Build history of the part. All positions in model axes, mm. Give positions to 0.01 mm unless a question says otherwise; leave off trailing zeros. Loops run counter-clockwise (first coordinate to the right, second up) from the corner with the lowest first, then second, coordinate; pieces in that order, holes last. Notation, with made-up numbers: (45, -34.75) -> (81, -34.75) arc R28 cw to (81, 2.25) -> close; hole circle Ø1 at (-22.75, 80.5). An arc over 180 degrees is marked (long way). Answer as a JSON object with one key per item and string values. Group by question number.
from build123d import *

# Parameters (mm, degrees)
SKETCH1_W                 = 50
SKETCH1_H                 = 8
BOSS_EXTRUDE1_DEPTH       = 3
F_8_CLEARANCE_HOLE1_D     = 4.4958
F_8_CLEARANCE_HOLE1_DEPTH = 17
F_8_CLEARANCE_HOLE1_TIP   = 1.350674586


with BuildPart() as part:
    # Sketch1 → Boss-Extrude1 (new body)
    with BuildSketch(Plane(origin=(0, 0, 0), x_dir=(1, 0, 0), z_dir=(0, 1, 0))):
        with Locations((17.773632998, 0.313559322)):
            Rectangle(SKETCH1_W, SKETCH1_H)
    extrude(amount=BOSS_EXTRUDE1_DEPTH)

    # #8 Clearance Hole1
    with Locations(Plane(origin=(7.773632998, 3, -0.313559322), x_dir=(0, 0, 1), z_dir=(0, 1, 0))):
        with Locations((0, 0), (0, 20), (0, 10)):
            Hole(F_8_CLEARANCE_HOLE1_D / 2, depth=F_8_CLEARANCE_HOLE1_DEPTH)
            with Locations((0, 0, -(F_8_CLEARANCE_HOLE1_DEPTH + F_8_CLEARANCE_HOLE1_TIP / 2))):  # 118° drill point
                Cone(0, F_8_CLEARANCE_HOLE1_D / 2, F_8_CLEARANCE_HOLE1_TIP, mode=Mode.SUBTRACT)


solid = part.part
(1) Pin check, flat tip, straight feed: pin 1 (1 mm diameter, centred on x = 7.5, z = -1.5, fed in from -Y). Stop position of the tip, or through.
(2) Saw through at B-B on x = 6. List the corners of the cut face in (y, z).
(3) Probe line 1 along X through (y, z) = (0.7, -0.25); line 2 along X through (y, z) = (0.85, -2); line 3 along Z through (x, y) = (27.5, 1.35). List the from-to ranges inside material, lowest first. Write a range as [from, to].
(4) Saw through at A-A on z = -1.5. List the corners of the cut face in (x, y).
(5) Saw through at D-D on z = 1. List the corners of the cut face in (x, y).
(6) Pull direction Z, two halves, no side cores. Call faces 1 (the flat face through (17, 1, -4.314)), 2 (the cylindrical face through (5.58, 1.48, 0.17)), 3 (the flat face through (17, 1, 3.686)), 4 (the flat face through (17, 3, -3)): pulls with the +Z half, pulls with the -Z half, needs draft (parallel to the pull), parting line crosses it, or undercut.
(7) Saw through at C-C on y = 2.05. List the corners of the cut face in (x, z), plus the area to 3 significant figures.
Calculated:
{
 "1": {"pin 1": "passes through"},
 "2": {"outline": "(0, -4.31) -> (3, -4.31) -> (3, -1.69) -> (0, -1.69) -> close; (0, 1.07) -> (3, 1.07) -> (3, 3.69) -> (0, 3.69) -> close"},
 "3": {"line 1": "x = [-7.23, 5.53], [10.02, 15.53], [20.02, 25.53], [30.02, 42.77]", "line 2": "x = [-7.23, 6.29], [9.26, 16.29], [19.26, 26.29], [29.26, 42.77]", "line 3": "z = [-4.31, -2.54], [1.92, 3.69]"},
 "4": {"outline": "(-7.23, 0) -> (5.86, 0) -> (5.86, 3) -> (-7.23, 3) -> close; (9.68, 0) -> (15.86, 0) -> (15.86, 3) -> (9.68, 3) -> close; (19.68, 0) -> (25.86, 0) -> (25.86, 3) -> (19.68, 3) -> close; (29.68, 0) -> (42.77, 0) -> (42.77, 3) -> (29.68, 3) -> close"},
 "5": {"outline": "(-7.23, 0) -> (5.95, 0) -> (5.95, 3) -> (-7.23, 3) -> close; (9.6, 0) -> (15.95, 0) -> (15.95, 3) -> (9.6, 3) -> close; (19.6, 0) -> (25.95, 0) -> (25.95, 3) -> (19.6, 3) -> close; (29.6, 0) -> (42.77, 0) -> (42.77, 3) -> (29.6, 3) -> close"},
 "6": {"face 1": "pulls with the -Z half", "face 2": "undercut", "face 3": "pulls with the +Z half", "face 4": "needs draft"},
 "7": {"outline": "(-7.23, -4.31) -> (42.77, -4.31) -> (42.77, 3.69) -> (-7.23, 3.69) -> close; hole circle Ø4.5 at (7.77, -0.31); hole circle Ø4.5 at (17.77, -0.31); hole circle Ø4.5 at (27.77, -0.31)", "area": "352 mm^2"}
}
